The drawing under review shows one solid part. Ordinate dimensions are in mm from its lowest x, y, z. Coordinates: 2 decimals unless noted, no trailing zeros. Write each loop counter-clockwise with the first axis right and the second up, starting at its lowest first coordinate (ties: lowest second). Pieces come first, ordered by that corner, then holes. Notation, with made-up numbers: M -28,2.5 L -18,2.5 A18 cw -18,31.5 Z; hole C 49.25,33 d9. An arc over 180 degrees is marked long. Write item = value, one per line.
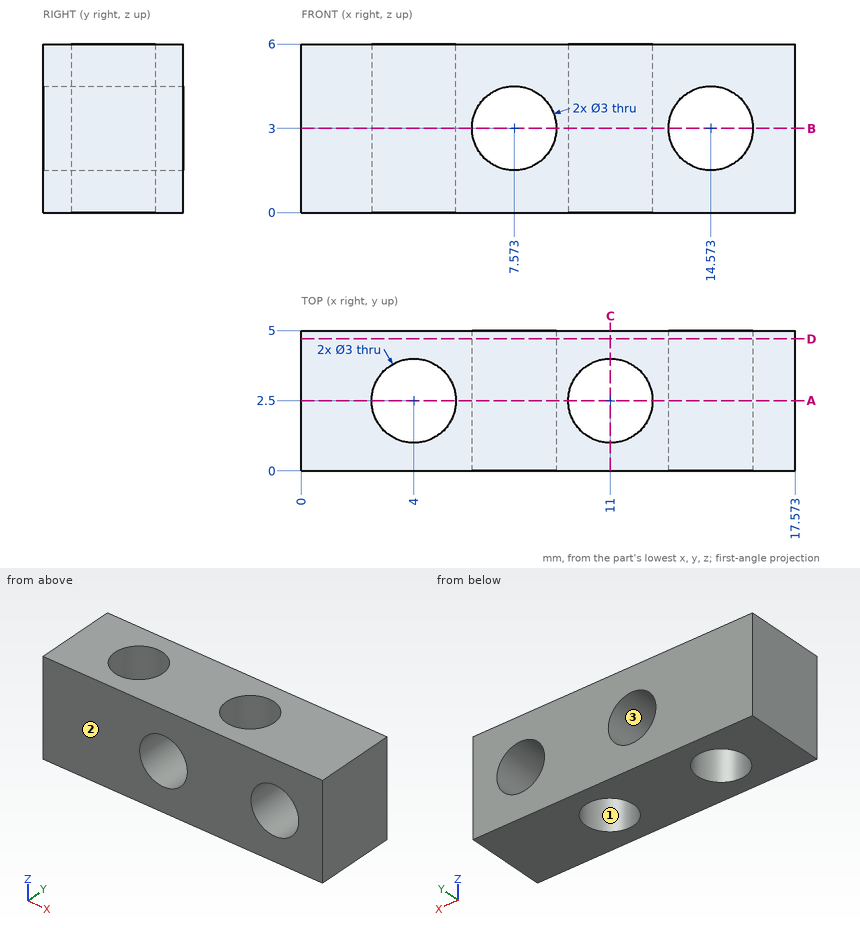
Q1. Consider section C-C, the plane x = 11. State the section outline as (y, z) points.
Check result:
outline = M 0,0 L 1,0 L 1,6 L 0,6 Z; M 4,0 L 5,0 L 5,6 L 4,6 Z
Q2. The part is to be moulded in two halves that separate along Y. For the marked faces 1, 2 and 3, say which applies: +Y half, -Y half, draft (parallel to the pull), parting line (faces both ways), or undercut.
Check result:
face_1 = undercut
face_2 = -Y half
face_3 = draft
Q3. Consider section B-B, the plane z = 3. State the section outline as (x, y) points.
Check result:
outline = M 0,0 L 6.07,0 L 6.07,5 L 0,5 Z; M 9.07,0 L 13.07,0 L 13.07,5 L 9.07,5 Z; M 16.07,0 L 17.57,0 L 17.57,5 L 16.07,5 Z; hole C 4,2.5 d3; hole C 11,2.5 d3
Q4. Consider section A-A, the plane y = 2.5. State the section outline as (x, z) points, and give its area (3 significant figures).
Check result:
outline = M 0,0 L 2.5,0 L 2.5,6 L 0,6 Z; M 5.5,0 L 9.5,0 L 9.5,6 L 5.5,6 Z; M 12.5,0 L 17.57,0 L 17.57,6 L 12.5,6 Z; hole C 7.57,3 d3; hole C 14.57,3 d3
area = 55.3 mm²
Q5. Wall thickness on line 1 (Y direction, x = 4, z = 4.1); line 2 (X direction, y = 2.15, z = 3); line 3 (X direction, y = 2.5, z = 1.65) (1 decimal): over which ranges is each line inside the solid? List them lowest first.
Check result:
line_1 = 0 to 1, 4 to 5
line_2 = 0 to 2.54, 5.46 to 6.07, 9.07 to 9.54, 12.46 to 13.07, 16.07 to 17.57
line_3 = 0 to 2.5, 5.5 to 6.9, 8.2 to 9.5, 12.5 to 13.9, 15.2 to 17.6
Q6. Consider section D-D, the plane y = 4.7. State the section outline as (x, z) points, and give its area (3 significant figures).
Check result:
outline = M 0,0 L 17.57,0 L 17.57,6 L 0,6 Z; hole C 7.57,3 d3; hole C 14.57,3 d3
area = 91.3 mm²
